Read the model definition and answer for the solid it produces. Units are mm, in the model's axes. A direction names the side the tool comes from. Round coordinates to 2 decimals unless told otherwise and drop trailing zeros. Write each loop counter-clockwise with the first axis right and the second up, starting at its lowest first coordinate (ties: lowest second). Pieces come first, ordered by that corner, then holes.
Autodesk Inventor part; units mm, degrees
ref_plane "Start Plane" through (0, 0, 0) normal (0, 0, 1) x (1, 0, 0)
ref_plane "End Plane" through (0, 0, 140) normal (0, 0, 1) x (1, 0, 0)
ref_plane "Work Plane5" through (-7, -100, 140) normal (0, 0, 1) x (1, 0, 0)
ref_plane "Start Plane" through (0, 0, 0) normal (0, 0, 1) x (1, 0, 0)
ref_plane "End Plane" through (0, 0, 140) normal (0, 0, 1) x (1, 0, 0)
sketch "Sketch" plane through (0, 0, 0) normal (0, 0, 1) x (1, 0, 0)
  line L0 (-10, -7) -> (-10, 7)
  line L1 (-7, 10) -> (7, 10)
  line L2 (10, 7) -> (10, -7)
  line L3 (7, -10) -> (-7, -10)
  arc A0 (-10, -7) -> (-7, -10) centre (-7, -7) ccw
  arc A1 (-7, 10) -> (-10, 7) centre (-7, 7) ccw
  arc A2 (10, 7) -> (7, 10) centre (7, 7) ccw
  arc A3 (7, -10) -> (10, -7) centre (7, -7) ccw
  arc A4 (-7, 8) -> (-8, 7) centre (-7, 7) ccw
  line L4 (-7, 8) -> (7, 8)
  arc A5 (8, 7) -> (7, 8) centre (7, 7) ccw
  line L5 (8, 7) -> (8, -7)
  arc A6 (7, -8) -> (8, -7) centre (7, -7) ccw
  line L6 (7, -8) -> (-7, -8)
  arc A7 (-8, -7) -> (-7, -8) centre (-7, -7) ccw
  line L7 (-8, -7) -> (-8, 7)
  line L8 (0, 14.8698) -> (0, -14.8698) construction
  line L9 (-14.8698, 0) -> (14.8698, 0) construction
  dimension "d7" = 3
  dimension "d10" = 20
  dimension "d11" = 20
  dimension "d12" = 2
  dimension "d15" = 10
  dimension "d16" = 10
extrude "Body" add sketch "Sketch" along normal up to surface (140 mm away) from surface at 0
sketch "Sketch3" plane through (0, 0, 0) normal (0, 0, 1) x (1, 0, 0)
  line L0 (0, 0) -> (10, 0)
ref_plane "Work Plane3" through (0, 0, 0) normal (0, -1, 0) x (1, 0, 0)
sketch "Sketch4" plane through (0, 0, 0) normal (0, -1, 0) x (1, 0, 0)
  line L0 (-2, 0) -> (12, 0)
  line L1 (-2, 140) -> (12, 140)
  dimension "d18" = 140
ref_plane "Work Plane5" through (-7, -100, 140) normal (0, 0, 1) x (1, 0, 0)
split "Split2" plane through (-7, -100, 140) removes the side toward (0, 0, 1)
equation "\"d7\" = G_IR"
equation "\"d10\" = G_H"
equation "\"d11\" = G_W"
equation "\"d12\" = G_T"
equation "\"d15\" = 0.5 * d10"
equation "\"d16\" = 0.5 * d11"
equation "\"d3\" = G_L"
equation "\"G_W\" = 20"
equation "\"G_H\" = 20"
equation "\"G_T\" = 2"
equation "\"G_IR\" = 3"
equation "\"G_L\" = d18"
equation "\"G_OFFSET_START\" = 0"
properties part number "ISO 12633-2 - 20x20x2 - 140" material "Steel, Mild"
Q1. Section A-A (z = 15) is taken. Determine the outline of the cut face in (x, y).
Verdict:
outline: (-10, -7) arc R3 ccw to (-7, -10) - (7, -10) arc R3 ccw to (10, -7) - (10, 7) arc R3 ccw to (7, 10) - (-7, 10) arc R3 ccw to (-10, 7) - close; hole (-8, -7) arc R1 ccw to (-7, -8) - (7, -8) arc R1 ccw to (8, -7) - (8, 7) arc R1 ccw to (7, 8) - (-7, 8) arc R1 ccw to (-8, 7) - close
Q2. Which of the six approach directions +Z, -Z, +X, -X, +Y, -Y give full straight-line access (tool end or side, diameter ignored) to faces 1 (the flat face through (8, 0, 69)), 2 (the flat face through (-9, 0, 0))?
Verdict:
face 1: +Z, -Z
face 2: -Z, +X, -X, +Y, -Y
Q3. Section B-B (x = 4.75) is taken. Determine the outline of the cut face in (y, z).
Verdict:
outline: (-10, 0) - (-8, 0) - (-8, 140) - (-10, 140) - close; (8, 0) - (10, 0) - (10, 140) - (8, 140) - close
Q4. Straight lines are drawn through the part: probe 1 along Y at (x, z) = (-5.75, 15); probe 2 along X at (y, z) = (7.5, 65.5). For each, find the intervals that lie inside material, in ascending order.
Verdict:
probe 1: y = -10 to -8, 8 to 10
probe 2: x = -9.96 to -7.87, 7.87 to 9.96
Q5. Determine the mould class of faces 3 (the flat face through (-9, 0, 140)), 4 (the cylindrical face through (9.1, 9.14, 69.02)), 5 (the flat face through (0, -8, 69)), 6 (the flat face through (0, -10, 69)) for opening direction Y: pulls with the +Y half, pulls with the -Y half, needs draft (parallel to the pull), parting line crosses it, or undercut.
Verdict:
face 3: needs draft
face 4: pulls with the +Y half
face 5: undercut
face 6: pulls with the -Y half
Q6. A flat-ended cylindrical pin translates along its axis: pin 1 Ø8 at (x, y) = (7, -0.5) entering from -Z. Find the tip coordinate at first contact, or state that the pin passes through.
Verdict:
pin 1: stops at z = 0
